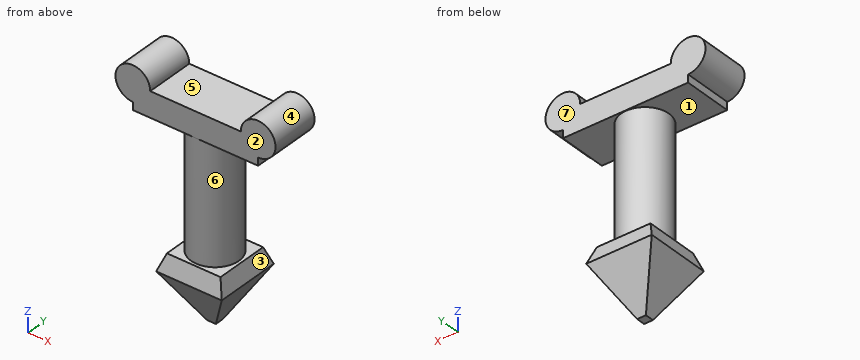
from build123d import *

# Parameters (mm, degrees)
F0_W      = 50.8
F0_H      = 50.8
F1_DEPTH  = 38.1
F1_TAPER  = 30
F1_FACE_W = 50.8
F1_FACE_H = 50.8
F2_DEPTH  = 12.7
F2_TAPER  = 20
F3_R      = 18.5436929907
F4_DEPTH  = 101.6
F6_DEPTH  = 19.05


with BuildPart() as f1:
    # F0 (on Top) → F1 (new body)
    with BuildSketch(Plane.XY):
        Rectangle(F0_W, F0_H)
    extrude(amount=-F1_DEPTH, taper=F1_TAPER)

    # F1_face (on face) → F2 (join)
    with BuildSketch(Plane.XY):
        Rectangle(F1_FACE_W, F1_FACE_H)
    extrude(amount=F2_DEPTH, taper=F2_TAPER)

    # F3 (on face) → F4 (join)
    with BuildSketch(Plane.XY.offset(12.7)):
        Circle(F3_R)
    extrude(amount=F4_DEPTH)

    # F5 (on Front) → F6 (join, symmetric)
    with BuildSketch(Plane.XZ):
        with BuildLine():
            ThreePointArc((48.5590323806, 111.0507363485), (58.0872045338, 134.0537787855), (35.0841620969, 124.5256066322))
            Line((35.0841620969, 124.5256066322), (-35.0841620969, 124.5256066322))
            ThreePointArc((-35.0841620969, 124.5256066322), (-58.0872045338, 134.0537787855), (-48.5590323806, 111.0507363485))
            Line((-48.5590323806, 111.0507363485), (-48.5590323806, 105.0193756819))
            Line((-48.5590323806, 105.0193756819), (48.5590323806, 105.0193756819))
            Line((48.5590323806, 105.0193756819), (48.5590323806, 111.0507363485))
        make_face()
    extrude(amount=F6_DEPTH, both=True)


solid = f1.part
Read the model definition and answer for the solid it produces. Units are mm, in the model's axes. Face numbers are marked on the shaded views. A direction names the side the tool comes from. Round coordinates to 2 decimals unless told otherwise and drop trailing zeros. Write each loop counter-clockwise with the first axis right and the second up, starting at its lowest first coordinate (ties: lowest second). Pieces come first, ordered by that corner, then holes. Notation, with made-up numbers: (30, 26.5) - (66, 26.5) arc R15 ccw to (66, 54.5) - close; hole circle Ø3 at (-35, 39.25). An arc over 180 degrees is marked (long way). One line per question, with ' | ' between items. Start each with the question number.
1. Each of these flat-tipped pins is pushed along its axis until it touches: pin 1 (3 mm diameter, centred on y = -6, z = 107.5, fed in from +X); pin 2 (6 mm diameter, centred on x = -42, y = -6.5, fed in from +Z); pin 3 (12 mm diameter, centred on y = 4, z = 95, fed in from -X); pin 4 (12 mm diameter, centred on x = -31, z = 98, fed in from +Y). Where does it stop, or does it pass through?
2. Section B-B (x = -41) is taken. Determine the outline of the cut face in (y, z), and give its area (3 significant figures).
3. Find the intervals of material crossed by probe 1 along Y at (x, z) = (-24, 117); probe 2 along Z at (x, y) = (-19, 13.5); probe 3 along Z at (x, y) = (17, -18), in increasing order. Write a range as [from, to].
4. Section A-A (z = 82.5) is taken. Determine the outline of the cut face in (x, y), and give its area (3 significant figures).
5. For a pull along Z with two mould halves and no side action, classify the marked faces 1, 2, 3 and 4 as +Z half, -Z half, draft (parallel to the pull), parting line (faces both ways), or undercut.
6. Section C-C (z = 122) is taken. Determine the outline of the cut face in (x, y), and give its area (3 significant figures).
7. For the marked faces 5, 6 and 7, determine the directions among +Z, -Z, +X, -X, +Y, -Y from which every point of the face is accessible in a straight line to the end or side of a thin tool.
Filled in:
1) pin 1: x = 48.56 | pin 2: z = 137.52 | pin 3: x = -18.54 | pin 4: through
2) outline: (-19.05, 105.02) - (19.05, 105.02) - (19.05, 135.68) - (-19.05, 135.68) - close | area: 1,170 mm²
3) probe 1: [-19.05, 19.05] | probe 2: [-11.09, 12.7], [105.02, 124.53] | probe 3: [-12.82, 12.7], [105.02, 124.53]
4) outline: circle Ø37.09 at (0, 0) | area: 1,080 mm²
5) face 1: undercut | face 2: draft | face 3: undercut | face 4: parting line
6) outline: (-61.8, -19.05) - (61.8, -19.05) - (61.8, 19.05) - (-61.8, 19.05) - close | area: 4,710 mm²
7) face 5: +Z, +Y, -Y | face 6: none | face 7: +Z, +X, -X, +Y
